from build123d import *

# Parameters (mm, degrees)
F2_DEPTH = 50.8
F3_W     = 45.810133
F3_H     = 19.05
F4_DEPTH = 50.8


with BuildPart() as f2:
    # F0 (on Front) → F2 (new body)
    with BuildSketch(Plane.XZ):
        with BuildLine():
            ThreePointArc((31.75, 19.05), (28.030256, 28.030256), (19.05, 31.75))
            Line((19.05, 31.75), (-19.05, 31.75))
            ThreePointArc((-19.05, 31.75), (-28.030256, 28.030256), (-31.75, 19.05))
            Line((-31.75, 19.05), (-31.75, -19.05))
            ThreePointArc((-31.75, -19.05), (-28.030256, -28.030256), (-19.05, -31.75))
            Line((-19.05, -31.75), (19.05, -31.75))
            ThreePointArc((19.05, -31.75), (28.030256, -28.030256), (31.75, -19.05))
            Line((31.75, -19.05), (31.75, 19.05))
        make_face()
        with BuildLine():
            ThreePointArc((19.05, 25.4), (23.540128, 23.540128), (25.4, 19.05))
            Line((25.4, 19.05), (25.4, -19.05))
            ThreePointArc((25.4, -19.05), (23.540128, -23.540128), (19.05, -25.4))
            Line((19.05, -25.4), (-19.05, -25.4))
            ThreePointArc((-19.05, -25.4), (-23.540128, -23.540128), (-25.4, -19.05))
            Line((-25.4, -19.05), (-25.4, 19.05))
            ThreePointArc((-25.4, 19.05), (-23.540128, 23.540128), (-19.05, 25.4))
            Line((-19.05, 25.4), (19.05, 25.4))
        make_face(mode=Mode.SUBTRACT)
    extrude(amount=F2_DEPTH)

    # F3 (on Front) → F4 (join)
    with BuildSketch(Plane.XZ):
        with Locations((23.405067, 41.275)):
            Rectangle(F3_W, F3_H)
    extrude(amount=F4_DEPTH)


solid = f2.part
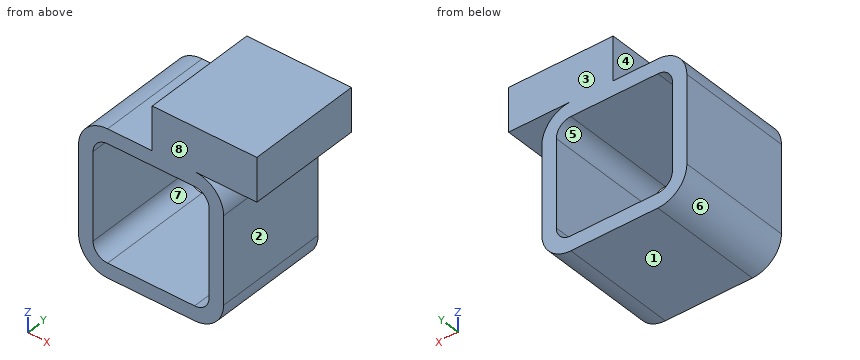
Input: part model. Units: mm. Frame: model coordinates. Face numbers are marked on the shaded views. A direction names the side the tool comes from. Round coordinates to 2 decimals unless told otherwise and drop trailing zeros. Order: outer loops, then holes, each group sorted by start corner. A loop starts at its lowest first (then second) coordinate and runs counter-clockwise, first axis right, second up.
1. Material intervals for line 1 (Z direction, x = 11, y = -24.5); line 2 (X direction, y = -13.5, z = 11), sorted ascending.
The answers:
line 1: z = -31.75 to -25.4, 25.4 to 50.8
line 2: x = -31.75 to -25.4, 25.4 to 31.75
2. Pin query (flat end, axial travel): P1, Ø6, axis at x = -6, y = -18, coming from the +Z side; P2, Ø15, axis at y = -33, z = 42.5, coming from the -X side; P3, Ø11.5, axis at y = -28.5, z = -8, coming from the +X side. Return the tip coordinate at first contact, or that it passes through.
The answers:
P1: stops at z = 31.75
P2: stops at x = 0.5
P3: stops at x = 31.75
3. Cut plane B-B, the plane y = -45.5. Output: boundary loops of the cut face in (x, z), then the cut area to 3 significant figures.
The answers:
outline: (-31.75, -19.05) arc R12.7 ccw to (-19.05, -31.75) - (19.05, -31.75) arc R12.7 ccw to (31.75, -19.05) - (31.75, 19.05) arc R12.7 ccw to (19.05, 31.75) - (46.31, 31.75) - (46.31, 50.8) - (0.5, 50.8) - (0.5, 31.75) - (-19.05, 31.75) arc R12.7 ccw to (-31.75, 19.05) - close; hole (-25.4, -19.05) arc R6.35 ccw to (-19.05, -25.4) - (19.05, -25.4) arc R6.35 ccw to (25.4, -19.05) - (25.4, 19.05) arc R6.35 ccw to (19.05, 25.4) - (-19.05, 25.4) arc R6.35 ccw to (-25.4, 19.05) - close
area: 2,220 mm2
4. Cut plane D-D, the plane z = 35.5. Output: boundary loops of the cut face in (x, y).
The answers:
outline: (0.5, -50.8) - (46.31, -50.8) - (46.31, 0) - (0.5, 0) - close
5. Cut plane A-A, the plane x = 17. Output: boundary loops of the cut face in (y, z).
The answers:
outline: (-50.8, -31.75) - (0, -31.75) - (0, -25.4) - (-50.8, -25.4) - close; (-50.8, 25.4) - (0, 25.4) - (0, 50.8) - (-50.8, 50.8) - close
6. Set-up query: the marked faces 1, 2, 3, 4 and 5. Return all of +Z, -Z, +X, -X, +Y, -Y with unobstructed straight access to the full face (end or side cutting, diameter ignored); none if empty.
The answers:
face 1: -Z, +X, -X, +Y, -Y
face 2: -Z, +X, +Y, -Y
face 3: +Z, -Z, +X, -X, +Y
face 4: +Z, -X, +Y, -Y
face 5: +Y, -Y
7. Cut plane C-C, the plane z = 15.5. Output: boundary loops of the cut face in (x, y), then the cut area to 3 significant figures.
The answers:
outline: (-31.75, -50.8) - (-25.4, -50.8) - (-25.4, 0) - (-31.75, 0) - close; (25.4, -50.8) - (31.75, -50.8) - (31.75, 0) - (25.4, 0) - close
area: 645 mm2
8. Mould query, pull axis Z, two halves, no side actions, for the marked faces 6, 7 and 8. Classes: released by +Z, released by -Z, zero draft, split by the parting line, or undercut.
The answers:
face 6: released by -Z
face 7: undercut
face 8: zero draft
